from build123d import *

# Parameters (mm, degrees)
SKETCH1_W               = 101.6
SKETCH1_H               = 50.8
BOSS_EXTRUDE1_DEPTH     = 354.289954614
CUT_EXTRUDE1_DEPTH      = 362.500555934
CUT_EXTRUDE1_DEPTH_BACK = 362.500555934
CUT_EXTRUDE2_DEPTH      = 362.500555934
CUT_EXTRUDE2_DEPTH_BACK = 362.500555934
SKETCH3_W               = 12.7
SKETCH3_H               = 354.289954614


with BuildPart() as part:
    # Sketch1 → Boss-Extrude1 (new body)
    with BuildSketch(Plane.XY):
        Rectangle(SKETCH1_W, SKETCH1_H)
    extrude(amount=BOSS_EXTRUDE1_DEPTH)

    # Sketch2 → Cut-Extrude1 (cut, two sides: drawn at the far end of the back side and taken through both)
    with BuildSketch(Plane(origin=(0, 25.4, 0), x_dir=(1, 0, 0), z_dir=(0, 1, 0)).offset(-CUT_EXTRUDE1_DEPTH_BACK)):
        Polygon((-50.8, -322.885251713), (-50.8, -310.060441542), (-29.982501618, -312.986150141), (-31.75, -325.562554614), (-35.787372775, -354.289954614), (-50.8, -354.289954614), align=None)
    extrude(amount=CUT_EXTRUDE1_DEPTH + CUT_EXTRUDE1_DEPTH_BACK, mode=Mode.SUBTRACT)

    # Sketch3 → Cut-Extrude2 (cut, two sides: drawn at the far end of the back side and taken through both)
    with BuildSketch(Plane(origin=(0, 25.4, 0), x_dir=(1, 0, 0), z_dir=(0, 1, 0)).offset(-CUT_EXTRUDE2_DEPTH_BACK)):
        with Locations((44.45, -177.144977307)):
            Rectangle(SKETCH3_W, SKETCH3_H)
    extrude(amount=CUT_EXTRUDE2_DEPTH + CUT_EXTRUDE2_DEPTH_BACK, mode=Mode.SUBTRACT)


solid = part.part
Model file for the job. Use its own axes, mm. Round coordinates to 2 decimals unless told otherwise and drop trailing zeros. Order: outer loops, then holes, each group sorted by start corner. A loop starts at its lowest first (then second) coordinate and runs counter-clockwise, first axis right, second up.
(1) Pin check, flat tip, straight feed: pin 1 (1.5 mm diameter, centred on x = -27.5, y = -5.5, fed in from -Z). Stop position of the tip, or through.
(2) Band-saw the part on A-A (y = -3). List the corners of the cut face in (x, z), then the cut area to 3 significant figures.
(3) Drill centre lines: line 1 (X direction, y = -15.5, z = 325); line 2 (Z direction, x = -36.5, y = -16.5). Where is each one in solid material? Low to high.
(4) Pull direction Z, two halves, no side cores. Call faces 1 (the face through (1, 0, 354.29)), 2 (the face through (-40.537, -0.356, 311.503)), 3 (the face through (-50.8, 0, 153)): released by +Z, released by -Z, zero draft, split by the parting line, or undercut.
(5) Band-saw the part on B-B (z = 332). List the corners of the cut face in (x, y), then the cut area to 3 significant figures.
Verdict:
1. pin 1: stops at z = 0
2. outline: (-50.8, 0) - (38.1, 0) - (38.1, 354.29) - (-35.79, 354.29) - (-29.98, 312.99) - (-50.8, 310.06) - close
2. area: 30,700 mm2
3. line 1: x = -31.67 to 38.1
3. line 2: z = 0 to 312.07
4. face 1: released by +Z
4. face 2: undercut
4. face 3: zero draft
5. outline: (-32.65, -25.4) - (38.1, -25.4) - (38.1, 25.4) - (-32.65, 25.4) - close
5. area: 3,590 mm2
